For this review, take the finished solid that the model builds, in its own axes (mm). Give positions to 0.01 mm unless a question says otherwise; leave off trailing zeros. Order: outer loops, then holes, each group sorted by start corner. A loop starts at its lowest first (then second) coordinate and runs counter-clockwise, first axis right, second up. Notation, with made-up numbers: (52, 71) - (99, 71) arc R9 ccw to (99, 75) - close; hole circle Ø10 at (44.25, 61). An arc over 180 degrees is marked (long way). Put each result on its own line as item: value. Start each with the question number.
```python
from build123d import *

# Parameters (mm, degrees)
BOSS_EXTRUDE1_DEPTH = 1.5
BOSS_EXTRUDE2_DEPTH = 1
SKETCH4_R           = 4.75
CUT_EXTRUDE1_DEPTH  = 23.898325822
SKETCH5_W           = 17.56
SKETCH5_H           = 2.5
BOSS_EXTRUDE3_DEPTH = 0.15


with BuildPart() as part:
    # Sketch1 → Boss-Extrude1 (new body)
    with BuildSketch(Plane.XY):
        with BuildLine():
            ThreePointArc((14.980604809, 6.55), (8.78, 2), (2.579395191, 6.55))
            Line((2.579395191, 6.55), (0, 6.55))
            Line((0, 6.55), (0, 0))
            Line((0, 0), (17.56, 0))
            Line((17.56, 0), (17.56, 6.55))
            Line((17.56, 6.55), (14.980604809, 6.55))
        make_face()
        with BuildLine():
            ThreePointArc((2.579395191, 6.55), (2.679421093, 10.743420825), (5.32, 14.002581212))
            Line((5.32, 14.002581212), (5.32, 14.619498126))
            ThreePointArc((5.32, 14.619498126), (1.449679407, 11.382680416), (0, 6.55))
            Line((0, 6.55), (2.579395191, 6.55))
        make_face()
        with BuildLine():
            ThreePointArc((12.24, 14.002581212), (14.880578907, 10.743420825), (14.980604809, 6.55))
            Line((14.980604809, 6.55), (17.56, 6.55))
            ThreePointArc((17.56, 6.55), (16.110320593, 11.382680416), (12.24, 14.619498126))
            Line((12.24, 14.619498126), (12.24, 14.002581212))
        make_face()
    extrude(amount=BOSS_EXTRUDE1_DEPTH)

    # Sketch3 → Boss-Extrude2 (add)
    with BuildSketch(Plane.XY.offset(1.5)):
        with BuildLine():
            Line((12.24, 14.619498126), (12.24, 14.002581212))
            ThreePointArc((12.24, 14.002581212), (8.78, 2), (5.32, 14.002581212))
            Line((5.32, 14.002581212), (5.32, 14.619498126))
            ThreePointArc((5.32, 14.619498126), (1.449679407, 11.382680416), (0, 6.55))
            Line((0, 6.55), (0, 0))
            Line((0, 0), (17.56, 0))
            Line((17.56, 0), (17.56, 6.55))
            ThreePointArc((17.56, 6.55), (16.110320593, 11.382680416), (12.24, 14.619498126))
        make_face()
        with BuildLine():
            Line((5.32, 14.619498126), (12.24, 14.619498126))
            Line((12.24, 14.619498126), (12.24, 14.002581212))
            ThreePointArc((12.24, 14.002581212), (8.78, 2), (5.32, 14.002581212))
            Line((5.32, 14.002581212), (5.32, 14.619498126))
        make_face()
    extrude(amount=BOSS_EXTRUDE2_DEPTH)

    # Sketch4 → Cut-Extrude1 (cut, through all)
    with BuildSketch(Plane(origin=(0, 0, 1.5), x_dir=(-1, 0, 0), z_dir=(0, 0, -1))):
        with Locations((-8.78, 8.5)):
            Circle(SKETCH4_R)
    extrude(amount=-CUT_EXTRUDE1_DEPTH, mode=Mode.SUBTRACT)

    # Sketch5 → Boss-Extrude3 (add)
    with BuildSketch(Plane.XZ):
        with Locations((8.78, 1.25)):
            Rectangle(SKETCH5_W, SKETCH5_H)
    extrude(amount=BOSS_EXTRUDE3_DEPTH)


solid = part.part
```
1. Clearance check with flat-ended pins moving along their axes: pin 1 (3 mm diameter, centred on x = 11, y = 12.5, fed in from -Z); pin 2 (2 mm diameter, centred on x = 10.5, y = 5.5, fed in from -Z); pin 3 (3 mm diameter, centred on x = 12.5, y = 3.5, fed in from -Z); pin 4 (0.7 mm diameter, centred on y = 14, z = 0.5, fed in from -X). State where each tip first meets the part, or that it passes through.
2. Add section D-D, the plane y = 8.5. Give the boundary of the cut face in (x, z).
3. Add section A-A, the plane x = 8.78. Give the boundary of the cut face in (y, z), then the cut area to 3 significant figures.
4. Add section C-C, the plane z = 0.35. Give the boundary of the cut face in (x, y).
5. Add section B-B, the plane z = 2.05. Give the boundary of the cut face in (x, y).
6. Wall thickness on line 1 (Y direction, x = 8.78, z = 1.8); line 2 (Z direction, x = 12, y = 4.25); line 3 (X direction, y = 12.75, z = 0.8): over which ranges is each line inside the solid? List them lowest first. Write a range as from..to.
7. The part is to be moulded in two halves that separate along Y. For faces 1 (the face through (12, 13, 1.5)), 2 (the face through (17.56, 3, 1)), 3 (the face through (16.15, 11.32, 1.23)), say which applies: released by +Y, released by -Y, zero draft, split by the parting line, or undercut.
Found:
1. pin 1: stops at z = 1.5
1. pin 2: passes through
1. pin 3: stops at z = 0
1. pin 4: stops at x = 3.61
2. outline: (0.22, 0) - (2.28, 0) - (2.28, 1.5) - (4.03, 1.5) - (4.03, 2.5) - (0.22, 2.5) - close; (13.53, 1.5) - (15.28, 1.5) - (15.28, 0) - (17.34, 0) - (17.34, 2.5) - (13.53, 2.5) - close
3. outline: (-0.15, 0) - (2, 0) - (2, 1.5) - (3.75, 1.5) - (3.75, 2.5) - (-0.15, 2.5) - close; (13.25, 1.5) - (14.62, 1.5) - (14.62, 2.5) - (13.25, 2.5) - close
3. area: 8.49 mm^2
4. outline: (0, -0.15) - (17.56, -0.15) - (17.56, 6.55) arc R8.78 ccw to (12.24, 14.62) - (12.24, 14) arc R6.5 cw (long way) to (5.32, 14) - (5.32, 14.62) arc R8.78 ccw to (0, 6.55) - close
5. outline: (0, -0.15) - (17.56, -0.15) - (17.56, 6.55) arc R8.78 ccw to (12.24, 14.62) - (5.32, 14.62) arc R8.78 ccw to (0, 6.55) - close; hole circle Ø9.5 at (8.78, 8.5)
6. line 1: y = -0.15..3.75, 13.25..14.62
6. line 2: z = 1.5..2.5
6. line 3: x = 2.56..3.86, 13.7..15
7. face 1: undercut
7. face 2: zero draft
7. face 3: released by +Y
